Check sheet for the modelled part. Datum: model origin and axes. Units: mm. A direction names the side the tool comes from. Round coordinates to 2 decimals unless told otherwise and drop trailing zeros. Loops run counter-clockwise (first coordinate to the right, second up) from the corner with the lowest first, then second, coordinate; pieces in that order, holes last. Notation, with made-up numbers: (77, 57.5) - (89, 57.5) arc R26 cw to (89, 88.5) - close; hole circle Ø9 at (34, 1.5). An arc over 180 degrees is marked (long way). Put each result on its own line as item: value.
```python
from build123d import *

# Parameters (mm, degrees)
F0_R     = 6.35
F1_DEPTH = 25.4
F2_R     = 5.55625
F3_DEPTH = 1.5875
F4_R     = 6.35
F5_DEPTH = 1.5875
F6_R     = 5.55625
F7_DEPTH = 1.5875
F8_R     = 6.35
F9_DEPTH = 1.5875


with BuildPart() as f1:
    # F0 (on Front) → F1 (new body)
    with BuildSketch(Plane.XZ):
        Circle(F0_R)
    extrude(amount=F1_DEPTH)

    # F2 (on face) → F3 (join)
    with BuildSketch(Plane.XZ.offset(25.4)):
        Circle(F2_R)
    extrude(amount=F3_DEPTH)

    # F4 (on face) → F5 (join)
    with BuildSketch(Plane.XZ.offset(26.9875)):
        Circle(F4_R)
    extrude(amount=F5_DEPTH)

    # F6 (on face) → F7 (join)
    with BuildSketch(Plane(origin=(0, 0, 0), x_dir=(-1, 0, 0), z_dir=(0, 1, 0))):
        Circle(F6_R)
    extrude(amount=F7_DEPTH)

    # F8 (on face) → F9 (join)
    with BuildSketch(Plane(origin=(0, 1.5875, 0), x_dir=(-1, 0, 0), z_dir=(0, 1, 0))):
        Circle(F8_R)
    extrude(amount=F9_DEPTH)


solid = f1.part
```
Item 1: Section check B-B on z = -5. Enter the section's corners in (x, y) (1 decimal), then the cut area to 3 significant figures.
Filled sheet:
outline: (-3.9, -28.6) - (3.9, -28.6) - (3.9, -27) - (2.4, -27) - (2.4, -25.4) - (3.9, -25.4) - (3.9, 0) - (2.4, 0) - (2.4, 1.6) - (3.9, 1.6) - (3.9, 3.2) - (-3.9, 3.2) - (-3.9, 1.6) - (-2.4, 1.6) - (-2.4, 0) - (-3.9, 0) - (-3.9, -25.4) - (-2.4, -25.4) - (-2.4, -27) - (-3.9, -27) - close
area: 239 mm²
Item 2: Section check C-C on y = -13. Enter the section's corners in (x, z).
Filled sheet:
outline: circle Ø12.7 at (0, 0)
Item 3: Thickness scan on line 1 (Y direction, x = 4, z = 4) (1 decimal); line 2 (X direction, y = -16.5, z = 3.5); line 3 (X direction, y = -13, z = -3). Record the ranges inside material, lowest first. Write a range as from..to.
Filled sheet:
line 1: -28.6..-27, -25.4..0, 1.6..3.2
line 2: -5.3..5.3
line 3: -5.6..5.6
Item 4: Go/stop test with flat-tipped pins: pin 1 (2 mm diameter, centred on x = -2, y = -3, fed in from +Z); pin 2 (1.5 mm diameter, centred on y = -21.5, z = 3, fed in from +X). Record where each tip stops, or that it passes through.
Filled sheet:
pin 1: z = 6.27
pin 2: x = 5.94
Item 5: Tool access check on faces 1 (the cylindrical face through (1.38, 2.37, -6.2)), 2 (the flat face through (0, 0, -6)). Record the directions out of +Z, -Z, +X, -X, +Y, -Y that give a thin tool (end or side, any length) a straight path to the whole face; none if there is none.
Filled sheet:
face 1: +Y, -Y
face 2: none
Item 6: Section check A-A on x = -4.75. Enter the section's corners in (y, z) (1 decimal).
Filled sheet:
outline: (-28.6, -4.2) - (-27, -4.2) - (-27, -2.9) - (-25.4, -2.9) - (-25.4, -4.2) - (0, -4.2) - (0, -2.9) - (1.6, -2.9) - (1.6, -4.2) - (3.2, -4.2) - (3.2, 4.2) - (1.6, 4.2) - (1.6, 2.9) - (0, 2.9) - (0, 4.2) - (-25.4, 4.2) - (-25.4, 2.9) - (-27, 2.9) - (-27, 4.2) - (-28.6, 4.2) - close
Item 7: Release check for a two-part mould opening along Y. For faces 3 (the flat face through (0, -28.575, 0)), 4 (the flat face through (0, 3.175, 0)), 5 (the cylindrical face through (-5.3, 0.78, 1.67)), 6 (the cylindrical face through (-1.38, -12.52, -6.2)) record: +Y half, -Y half, draft (parallel to the pull), parting line (faces both ways), or undercut.
Filled sheet:
face 3: -Y half
face 4: +Y half
face 5: undercut
face 6: draft
